Source: CAD feature listing. Evaluate the final solid. Frame: model axes, mm. A direction names the side the tool comes from. Give positions to 0.01 mm unless a question says otherwise; leave off trailing zeros. Order: outer loops, then holes, each group sorted by start corner. A loop starts at its lowest first (then second) coordinate and runs counter-clockwise, first axis right, second up. Notation, with made-up numbers: (-16.75, 69) - (39.25, 69) arc R11 cw to (39.25, 76) - close; hole circle Ø11 at (36.25, 72). An arc over 180 degrees is marked (long way). Answer as CSV lines item,"result".
```python
from build123d import *

# Parameters (mm, degrees)
CUBE_W                    = 150
CUBE_H                    = 150
BOSS_EXTRU_1_DEPTH        = 34.5
PAVE_W                    = 96
PAVE_H                    = 144
ENL_V_MAT_EXTRU_1_DEPTH   = 31.5
VIS1_R                    = 2.5
ENL_V_MAT_EXTRU_2_DEPTH   = 5
ENL_V_START               = -5
VIS2_R                    = 2.5
ENL_V_MAT_EXTRU_3_DEPTH   = 5
PAVE_PROCHE_MOTEUR_W      = 12.5
PAVE_PROCHE_MOTEUR_H      = 124
ENL_V_MAT_EXTRU_4_DEPTH   = 31.5
PAVE_ROUE_LIBRE_W         = 32.86
PAVE_ROUE_LIBRE_H         = 15.696676457
PAVE_ROUE_LIBRE_H_2       = 18.419496328
ENL_V_MAT_EXTRU_5_DEPTH   = 36
CABLES_W                  = 22.36
CABLES_H                  = 10
ENL_V_MAT_EXTRU_6_DEPTH   = 36
ROUE_EXT_R                = 32
ENL_V_MAT_EXTRU_7_DEPTH   = 8
ROUE_INTER_R              = 16.02
ENL_V_MAT_EXTRU_8_DEPTH   = 69
ENL_V_START_2             = -7.5
ROUE_EXT2_R               = 32
ENL_V_MAT_EXTRU_9_DEPTH   = 7.5
ENL_V_START_3             = -69
ROUE_INTER2_R             = 16.02
ENL_V_MAT_EXTRU_10_DEPTH  = 69
VIS_MOTEUR_POUR_SUPPORT_R = 2.5
ENL_V_MAT_EXTRU_11_DEPTH  = 10
BOSS_EXTRU_2_DEPTH        = 10
ESQUISSE2_R               = 2.5
ENL_V_MAT_EXTRU_12_DEPTH  = 10
ESQUISSE3_W               = 3.439870431
ESQUISSE3_H               = 124
BOSS_EXTRU_3_DEPTH        = 31
ESQUISSE5_W               = 3.439870431
ESQUISSE5_H               = 124
BOSS_EXTRU_4_DEPTH        = 0.5
ESQUISSE6_R               = 2.5
ENL_V_MAT_EXTRU_13_DEPTH  = 10
ESQUISSE7_R               = 2.5
ENL_V_MAT_EXTRU_14_DEPTH  = 10
ESQUISSE8_R               = 2.5
ENL_V_MAT_EXTRU_15_DEPTH  = 10


with BuildPart() as part:
    # Cube → Boss.-Extru.1 (new body)
    with BuildSketch(Plane(origin=(0, 0, 0), x_dir=(1, 0, 0), z_dir=(0, 1, 0))):
        with Locations((-34.210526316, -11.513157895)):
            Rectangle(CUBE_W, CUBE_H)
    extrude(amount=BOSS_EXTRU_1_DEPTH)

    # Pave → Enlèv. mat.-Extru.1 (cut)
    with BuildSketch(Plane(origin=(0, 34.5, 0), x_dir=(1, 0, 0), z_dir=(0, 1, 0))):
        with Locations((-10.210526316, -11.513157895)):
            Rectangle(PAVE_W, PAVE_H)
    extrude(amount=-ENL_V_MAT_EXTRU_1_DEPTH, mode=Mode.SUBTRACT)

    # Vis1 → Enlèv. mat.-Extru.2 (cut)
    with BuildSketch(Plane.XY.offset(86.513157895)):
        with Locations((33.789473684, 10)):
            Circle(VIS1_R)
        with Locations((33.789473684, 20)):
            Circle(VIS1_R)
        with Locations((33.789473684, 30)):
            Circle(VIS1_R)
    extrude(amount=-ENL_V_MAT_EXTRU_2_DEPTH, mode=Mode.SUBTRACT)

    # Vis2 → Enlèv. mat.-Extru.3 (cut)
    with BuildSketch(Plane(origin=(0, 0, -63.486842105), x_dir=(-1, 0, 0), z_dir=(0, 0, -1)).offset(ENL_V_START)):
        with Locations(Location((-33.789473684, 10, 0), (0, 0, 180))):
            Circle(VIS2_R)
        with Locations(Location((-33.789473684, 20, 0), (0, 0, 180))):
            Circle(VIS2_R)
        with Locations(Location((-33.789473684, 30, 0), (0, 0, 180))):
            Circle(VIS2_R)
    extrude(amount=ENL_V_MAT_EXTRU_3_DEPTH, mode=Mode.SUBTRACT)

    # Pave proche moteur → Enlèv. mat.-Extru.4 (cut)
    with BuildSketch(Plane(origin=(0, 34.5, 0), x_dir=(1, 0, 0), z_dir=(0, 1, 0))):
        with Locations((-67.460526316, -11.513157895)):
            Rectangle(PAVE_PROCHE_MOTEUR_W, PAVE_PROCHE_MOTEUR_H)
    extrude(amount=-ENL_V_MAT_EXTRU_4_DEPTH, mode=Mode.SUBTRACT)

    # Pave Roue libre → Enlèv. mat.-Extru.5 (cut)
    with BuildSketch(Plane(origin=(0, 34.5, 0), x_dir=(1, 0, 0), z_dir=(0, 1, 0))):
        with Locations((-87.980526316, 61.335180334)):
            Rectangle(PAVE_ROUE_LIBRE_W, PAVE_ROUE_LIBRE_H)
        with Locations((-87.980526316, -85.722906059)):
            Rectangle(PAVE_ROUE_LIBRE_W, PAVE_ROUE_LIBRE_H_2)
    extrude(amount=-ENL_V_MAT_EXTRU_5_DEPTH, mode=Mode.SUBTRACT)

    # Cables → Enlèv. mat.-Extru.6 (cut)
    with BuildSketch(Plane(origin=(0, 34.5, 0), x_dir=(1, 0, 0), z_dir=(0, 1, 0))):
        with Locations((-89.710526316, -0.513157895)):
            Rectangle(CABLES_W, CABLES_H)
        with Locations((-89.710526316, -22.513157895)):
            Rectangle(CABLES_W, CABLES_H)
    extrude(amount=-ENL_V_MAT_EXTRU_6_DEPTH, mode=Mode.SUBTRACT)

    # Roue ext → Enlèv. mat.-Extru.7 (cut)
    with BuildSketch(Plane.XY.offset(86.513157895)):
        with Locations((-82.5, 10)):
            Circle(ROUE_EXT_R)
    extrude(amount=-ENL_V_MAT_EXTRU_7_DEPTH, mode=Mode.SUBTRACT)

    # Roue inter → Enlèv. mat.-Extru.8 (cut)
    with BuildSketch(Plane.XY.offset(86.513157895)):
        with Locations((-82.5, 10)):
            Circle(ROUE_INTER_R)
    extrude(amount=-ENL_V_MAT_EXTRU_8_DEPTH, mode=Mode.SUBTRACT)

    # Roue ext2 → Enlèv. mat.-Extru.9 (cut)
    with BuildSketch(Plane(origin=(0, 0, -63.486842105), x_dir=(-1, 0, 0), z_dir=(0, 0, -1)).offset(ENL_V_START_2)):
        with Locations((82.5, 10)):
            Circle(ROUE_EXT2_R)
    extrude(amount=ENL_V_MAT_EXTRU_9_DEPTH, mode=Mode.SUBTRACT)

    # Roue inter2 → Enlèv. mat.-Extru.10 (cut)
    with BuildSketch(Plane(origin=(0, 0, -63.486842105), x_dir=(-1, 0, 0), z_dir=(0, 0, -1)).offset(ENL_V_START_3)):
        with Locations((82.5, 10)):
            Circle(ROUE_INTER2_R)
    extrude(amount=ENL_V_MAT_EXTRU_10_DEPTH, mode=Mode.SUBTRACT)

    # Vis Moteur pour support → Enlèv. mat.-Extru.11 (cut)
    with BuildSketch(Plane(origin=(-58.210526316, 0, 0), x_dir=(0, 0, -1), z_dir=(1, 0, 0))):
        with Locations((-68.513157895, 8)):
            Circle(VIS_MOTEUR_POUR_SUPPORT_R)
        with Locations((-68.513157895, 18)):
            Circle(VIS_MOTEUR_POUR_SUPPORT_R)
        with Locations((-68.513157895, 28)):
            Circle(VIS_MOTEUR_POUR_SUPPORT_R)
        with Locations((45.986842105, 8)):
            Circle(VIS_MOTEUR_POUR_SUPPORT_R)
        with Locations((45.986842105, 18)):
            Circle(VIS_MOTEUR_POUR_SUPPORT_R)
        with Locations((45.986842105, 28)):
            Circle(VIS_MOTEUR_POUR_SUPPORT_R)
    extrude(amount=-ENL_V_MAT_EXTRU_11_DEPTH, mode=Mode.SUBTRACT)

    # Esquisse1 → Boss.-Extru.2 (add)
    with BuildSketch(Plane(origin=(0, 3, 0), x_dir=(1, 0, 0), z_dir=(0, 1, 0))):
        Polygon((-58.210526316, -15.513157895), (-14.210526316, -15.513157895), (-14.210526316, -83.513157895), (-6.210526316, -83.513157895), (-6.210526316, -15.513157895), (37.789473684, -15.513157895), (37.789473684, -7.513157895), (-6.210526316, -7.513157895), (-6.210526316, 60.486842105), (-14.210526316, 60.486842105), (-14.210526316, -7.513157895), (-58.210526316, -7.513157895), align=None)
    extrude(amount=BOSS_EXTRU_2_DEPTH)

    # Esquisse2 → Enlèv. mat.-Extru.12 (cut)
    with BuildSketch(Plane.XY.offset(15.513157895)):
        with Locations((-43.942882256, 8)):
            Circle(ESQUISSE2_R)
        with Locations((-26.88958752, 8)):
            Circle(ESQUISSE2_R)
        with Locations((9.588466595, 8)):
            Circle(ESQUISSE2_R)
        with Locations((23.56238511, 8)):
            Circle(ESQUISSE2_R)
    extrude(amount=-ENL_V_MAT_EXTRU_12_DEPTH, mode=Mode.SUBTRACT)

    # Esquisse3 → Boss.-Extru.3 (add)
    with BuildSketch(Plane(origin=(0, 3, 0), x_dir=(1, 0, 0), z_dir=(0, 1, 0))):
        with Locations((-62.930461532, -11.513157895)):
            Rectangle(ESQUISSE3_W, ESQUISSE3_H)
    extrude(amount=BOSS_EXTRU_3_DEPTH)

    # Esquisse5 → Boss.-Extru.4 (add)
    with BuildSketch(Plane(origin=(0, 34, 0), x_dir=(1, 0, 0), z_dir=(0, 1, 0))):
        with Locations((-62.930461532, -11.513157895)):
            Rectangle(ESQUISSE5_W, ESQUISSE5_H)
    extrude(amount=BOSS_EXTRU_4_DEPTH)

    # Esquisse6 → Enlèv. mat.-Extru.13 (cut)
    with BuildSketch(Plane(origin=(-58.210526316, 0, 0), x_dir=(0, 0, -1), z_dir=(1, 0, 0))):
        with Locations((-68.513157895, 28)):
            Circle(ESQUISSE6_R)
        with Locations((-68.513157895, 18)):
            Circle(ESQUISSE6_R)
        with Locations((-68.513157895, 8)):
            Circle(ESQUISSE6_R)
        with Locations((45.986842105, 28)):
            Circle(ESQUISSE6_R)
        with Locations((45.986842105, 18)):
            Circle(ESQUISSE6_R)
        with Locations((45.986842105, 8)):
            Circle(ESQUISSE6_R)
    extrude(amount=-ENL_V_MAT_EXTRU_13_DEPTH, mode=Mode.SUBTRACT)

    # Esquisse7 → Enlèv. mat.-Extru.14 (cut)
    with BuildSketch(Plane(origin=(-58.210526316, 0, 0), x_dir=(0, 0, -1), z_dir=(1, 0, 0))):
        with Locations((0, 8.527871685)):
            Circle(ESQUISSE7_R)
        with Locations((0, 18.750861141)):
            Circle(ESQUISSE7_R)
        with Locations((-25.400224022, 8.527871685)):
            Circle(ESQUISSE7_R)
        with Locations((-25.400224022, 18.750861141)):
            Circle(ESQUISSE7_R)
        with Locations((-50.386538843, 8.527871685)):
            Circle(ESQUISSE7_R)
        with Locations((23.629525814, 8.527871685)):
            Circle(ESQUISSE7_R)
    extrude(amount=-ENL_V_MAT_EXTRU_14_DEPTH, mode=Mode.SUBTRACT)

    # Esquisse8 → Enlèv. mat.-Extru.15 (cut)
    with BuildSketch(Plane(origin=(0, 3, 0), x_dir=(1, 0, 0), z_dir=(0, 1, 0))):
        with Locations(Location((19.789473684, -43.513157895, 0), (0, 0, 270))):
            Circle(ESQUISSE8_R)
        with Locations(Location((19.789473684, 20.486842105, 0), (0, 0, 270))):
            Circle(ESQUISSE8_R)
    extrude(amount=-ENL_V_MAT_EXTRU_15_DEPTH, mode=Mode.SUBTRACT)


solid = part.part
```
(1) Cut plane A-A (x = -82.5). Return loops of the section in (y, z).
Completed:
outline,"(0, 5.51) - (34.5, 5.51) - (34.5, 17.51) - (0, 17.51) - close; (26.02, -53.49) - (34.5, -53.49) - (34.5, -4.49) - (26.02, -4.49) - close; (26.02, 27.51) - (34.5, 27.51) - (34.5, 76.51) - (26.02, 76.51) - close"
(2) Cut plane B-B (x = 0.5). Return loops of the section in (y, z).
Completed:
outline,"(0, -63.49) - (34.5, -63.49) - (34.5, -60.49) - (3, -60.49) - (3, 7.51) - (13, 7.51) - (13, 15.51) - (3, 15.51) - (3, 83.51) - (34.5, 83.51) - (34.5, 86.51) - (0, 86.51) - close"
(3) Ray query, line 1 (Z direction, x = 18.5, y = 8.5); line 2 (Z direction, x = -83, y = 27); line 3 (Z direction, x = 27, y = 30). Return the intervals inside material, ascending. Write a range as from..to.
Completed:
line 1,"-63.49..-60.49, 7.51..15.51, 83.51..86.51"
line 2,"-53.49..-4.49, 5.51..17.51, 27.51..76.51"
line 3,"-63.49..-60.49, 83.51..86.51"
(4) Mould query, pull axis Z, two halves, no side actions, for faces 1 (the flat face through (-11, 19, 83.513)), 2 (the cylindrical face through (31.947, 28.31, -61.966)), 3 (the flat face through (-107, 33, -63.487)). Classes: released by +Z, released by -Z, zero draft, split by the parting line, or undercut.
Completed:
face 1,"undercut"
face 2,"zero draft"
face 3,"released by -Z"
(5) Access query for faces 4 (the cylindrical face through (-41.634, 7.042, 11.569)), 5 (the flat face through (15, 3, -27)), 6 (the cylindrical face through (-89.72, 24.3, 48.44)). Directions: +Z, -Z, +X, -X, +Y, -Y. A direction counts if a zero-diameter tool reaches every point of the face in a straight line with its end or side. Return the directions, or none.
Completed:
face 4,"none"
face 5,"+Y"
face 6,"+Z"
(6) Contact query for flat-ended pins moving along their axis: pin 1 (1.5 mm diameter, centred on x = -19, z = 69.5, fed in from +Y); pin 2 (10 mm diameter, centred on x = -60, y = 17.5, fed in from +Z); pin 3 (6.5 mm diameter, centred on x = -88, y = 12.5, fed in from -Z). Output: stop coordinate, or through.
Completed:
pin 1,"y = 3"
pin 2,"z = 78.51"
pin 3,"z = 5.51"
(7) Cut plane D-D (z = -13). Return loops of the section in (x, y), then the cut area to 3 significant figures.
Completed:
outline,"(-109.21, 0) - (-95.02, 0) arc R16.02 cw to (-73.71, 23.39) - (-73.71, 34.5) - (-109.21, 34.5) - close; (-69.98, 0) - (40.79, 0) - (40.79, 34.5) - (37.79, 34.5) - (37.79, 3) - (-6.21, 3) - (-6.21, 13) - (-14.21, 13) - (-14.21, 3) - (-58.21, 3) - (-58.21, 34.5) - (-64.65, 34.5) - (-64.65, 3) - (-68.09, 3) arc R16.02 cw to start"
area,"1,360 mm²"
(8) Cut plane C-C (z = 68). Give the number of separate pieces and of enclosed holes in the cut face, then the cut area to 3 significant figures.
Completed:
separate pieces,"5"
enclosed holes,"0"
area,"1,260 mm²"
